Design review of the part built by this model. Coordinates are the model's own, in mm. A direction names the side the tool comes from. Give positions to 0.01 mm unless a question says otherwise; leave off trailing zeros. Write each loop counter-clockwise with the first axis right and the second up, starting at its lowest first coordinate (ties: lowest second). Pieces come first, ordered by that corner, then holes. Notation, with made-up numbers: (87, 22.5) -> (117, 22.5) arc R19 cw to (117, 36.5) -> close; hole circle Ø1 at (59.25, 30). An arc over 180 degrees is marked (long way). Use CSV: the item, a comma, the result in double quotes.
```python
from build123d import *

# Parameters (mm, degrees)
SKETCH_1_W      = 5.15
SKETCH_1_H      = 5.025
EXTRUDE_1_DEPTH = 12
SKETCH_2_R      = 0.6
EXTRUDE_2_DEPTH = 11.6
SKETCH_3_R      = 16
EXTRUDE_3_DEPTH = 6.5


with BuildPart() as part:
    # 草图1 → 凸台-拉伸1 (new body)
    with BuildSketch(Plane(origin=(0, 0, 0), x_dir=(1, 0, 0), z_dir=(0, 1, 0))):
        Polygon((-10.125, 5.025), (-10.125, 0), (-10.125, -5.025), (15.275, -5.025), (15.275, 5.025), align=None)
        Polygon((-15.275, 12.975), (-15.275, 0), (-10.125, 0), (-10.125, 5.025), (-10.125, 12.975), align=None)
        with Locations((-12.7, -2.5125)):
            Rectangle(SKETCH_1_W, SKETCH_1_H)
    extrude(amount=EXTRUDE_1_DEPTH)

    # 草图2 → 凸台-拉伸2 (add)
    with BuildSketch(Plane(origin=(15.275, 0, 0), x_dir=(0, 0, -1), z_dir=(1, 0, 0))):
        with Locations(Location((0, 6, 0), (0, 0, 180))):
            Circle(SKETCH_2_R)
    extrude(amount=EXTRUDE_2_DEPTH)

    # 草图3 → 凸台-拉伸3 (add)
    with BuildSketch(Plane(origin=(26.875, 0, 0), x_dir=(0, 0, -1), z_dir=(1, 0, 0))):
        with Locations((0, 6)):
            Circle(SKETCH_3_R)
    extrude(amount=-EXTRUDE_3_DEPTH)


solid = part.part
```
(1) Mouldability with a two-part tool opening along X and no side actions: class faces 4 (the face through (26.875, 6, 0)), 5 (the face through (3, 6, -5.025)), 6 (the face through (0, 6, 5.025)) as +X half, -X half, draft (parallel to the pull), parting line (faces both ways), or undercut.
Established:
face 4,"+X half"
face 5,"undercut"
face 6,"draft"
(2) For line 1 along X through (y, z) = (6.5, -3.5) (3 decimals); line 2 along X through (y, z) = (9, -11) (3 decimals); line 3 along Z through (x, y) = (14.5, 9) (3 decimals), list the stretches that pass through material, from the lowest coordinate up. Write a range as [from, to].
Established:
line 1,"x = [-15.275, 15.275], [20.375, 26.875]"
line 2,"x = [-15.275, -10.125], [20.375, 26.875]"
line 3,"z = [-5.025, 5.025]"
(3) Tool access review of faces 1 (the face through (-10.125, 6, -9)), 2 (the face through (-4, 12, -2)), 3 (the face through (-4, 0, -2)): name each direction out of +Z, -Z, +X, -X, +Y, -Y from which nothing blocks a thin tool from reaching the whole face with its end or side.
Established:
face 1,"-Z, +Y, -Y"
face 2,"+Z, -Z, -X, +Y"
face 3,"+Z, -Z, -X, -Y"
(4) Clearance check with flat-ended pins moving along their axes: pin 1 (10 mm diameter, centred on x = 0.5, y = 11, fed in from +Z) (3 decimals); pin 2 (1 mm diameter, centred on y = -4.5, z = 10, fed in from -X) (3 decimals); pin 3 (1.5 mm diameter, centred on x = -13.5, y = 8.5, fed in from -Z) (3 decimals); pin 4 (1.5 mm diameter, centred on x = 11, z = 7, fed in from +Y). State where each tip first meets the part, or that it passes through.
Established:
pin 1,"stops at z = 5.025"
pin 2,"stops at x = 20.375"
pin 3,"stops at z = -12.975"
pin 4,"passes through"
(5) Take a section at B-B (y = 6). Write out the cut boundary in (x, z) (3 decimals), then the cut area to 3 significant figures.
Established:
outline,"(-15.275, -12.975) -> (-10.125, -12.975) -> (-10.125, -5.025) -> (15.275, -5.025) -> (15.275, -0.6) -> (20.375, -0.6) -> (20.375, -16) -> (26.875, -16) -> (26.875, 16) -> (20.375, 16) -> (20.375, 0.6) -> (15.275, 0.6) -> (15.275, 5.025) -> (-15.275, 5.025) -> close"
area,"562 mm2"
(6) Take a section at A-A (z = 2). Write out the cut boundary in (x, y) (1 decimal).
Established:
outline,"(-15.3, 0) -> (15.3, 0) -> (15.3, 12) -> (-15.3, 12) -> close; (20.4, -9.9) -> (26.9, -9.9) -> (26.9, 21.9) -> (20.4, 21.9) -> close"
(7) Take a section at C-C (x = 10). Write out the cut boundary in (y, z) (3 decimals).
Established:
outline,"(0, -5.025) -> (12, -5.025) -> (12, 5.025) -> (0, 5.025) -> close"
(8) Take a section at D-D (z = -3.5). Write out the cut boundary in (x, y) (1 decimal), then the cut area to 3 significant figures.
Established:
outline,"(-15.3, 0) -> (15.3, 0) -> (15.3, 12) -> (-15.3, 12) -> close; (20.4, -9.6) -> (26.9, -9.6) -> (26.9, 21.6) -> (20.4, 21.6) -> close"
area,"570 mm2"
